from build123d import *

# Parameters (mm, degrees)
ESQUISSE1_W             = 40
ESQUISSE1_H             = 70.5
BOSS_EXTRU_1_DEPTH      = 2
ESQUISSE2_R             = 10
ENL_V_MAT_EXTRU_1_DEPTH = 2
ESQUISSE3_R             = 6.03
ENL_V_MAT_EXTRU_2_DEPTH = 10


with BuildPart() as part:
    # Esquisse1 → Boss.-Extru.1 (new body)
    with BuildSketch(Plane(origin=(0, 0, 0), x_dir=(1, 0, 0), z_dir=(0, 1, 0))):
        with Locations((-5, 5.25)):
            Rectangle(ESQUISSE1_W, ESQUISSE1_H)
        with BuildLine():
            Line((-50, 40.5), (40, 40.5))
            ThreePointArc((40, 40.5), (-5, 85.5), (-50, 40.5))
        make_face()
    extrude(amount=BOSS_EXTRU_1_DEPTH)

    # Esquisse2 → Enlèv. mat.-Extru.1 (cut)
    with BuildSketch(Plane(origin=(0, 2, 0), x_dir=(1, 0, 0), z_dir=(0, 1, 0))):
        with Locations((-5, 40.5)):
            Circle(ESQUISSE2_R)
    extrude(amount=-ENL_V_MAT_EXTRU_1_DEPTH, mode=Mode.SUBTRACT)

    # Esquisse3 → Enlèv. mat.-Extru.2 (cut)
    with BuildSketch(Plane(origin=(0, 0, 0), x_dir=(-1, 0, 0), z_dir=(0, -1, 0))):
        with Locations((5, 75.5)):
            Circle(ESQUISSE3_R)
    extrude(amount=-ENL_V_MAT_EXTRU_2_DEPTH, mode=Mode.SUBTRACT)


solid = part.part
CAD build for the part. Positions are in the model's coordinates, mm. Round coordinates to 2 decimals unless told otherwise and drop trailing zeros. Write each loop counter-clockwise with the first axis right and the second up, starting at its lowest first coordinate (ties: lowest second). Pieces come first, ordered by that corner, then holes.
(1) Slice it at B-B, the plane x = -5. Write the cut outline in (y, z), and give its area (3 significant figures).
(2) Mould opens along X. For faces 1 (the face through (-7.17, 1.01, -30.74)), 2 (the face through (-4.01, 0.99, -85.49)), 3 (the face through (-6, 0, -29)) say: pulls with the +X half, pulls with the -X half, needs draft (parallel to the pull), parting line crosses it, or undercut.
(3) Probe line 1 along Z through (x, y) = (-5, 1); line 2 along Z through (x, y) = (-3.5, 0.75) (3 decimals); line 3 along X through (y, z) = (1.55, -75.5). List the from-to ranges inside material, lowest first.
(4) Slice it at D-D, the plane z = -15. Write the cut outline in (x, y).
(5) Slice it at C-C, the plane z = -75.5. Write the cut outline in (x, y).
(6) Slice it at A-A, the plane y = 1.6. Write the cut outline in (x, z).
(7) Drop flat-ended pins along their axis: P1, Ø1, axis at y = 0.5, z = 2.5, coming from the -X side; P2, Ø1, axis at y = 1.5, z = -73, coming from the +X side; P3, Ø1, axis at x = -38.5, y = 0.5, coming from the +Z side; P4, Ø19.5, axis at x = -5, z = -75.5, coming from the +Y side. Give the stop position or say it passes through.
From the geometry:
1. outline: (0, -85.5) - (2, -85.5) - (2, -81.53) - (0, -81.53) - close; (0, -69.47) - (2, -69.47) - (2, -50.5) - (0, -50.5) - close; (0, -30.5) - (2, -30.5) - (2, 30) - (0, 30) - close
1. area: 167 mm2
2. face 1: undercut
2. face 2: parting line crosses it
2. face 3: needs draft
3. line 1: z = -85.5 to -81.53, -69.47 to -50.5, -30.5 to 30
3. line 2: z = -85.475 to -81.34, -69.66 to -50.387, -30.613 to 30
3. line 3: x = -33.28 to -11.03, 1.03 to 23.28
4. outline: (-25, 0) - (15, 0) - (15, 2) - (-25, 2) - close
5. outline: (-33.28, 0) - (-11.03, 0) - (-11.03, 2) - (-33.28, 2) - close; (1.03, 0) - (23.28, 0) - (23.28, 2) - (1.03, 2) - close
6. outline: (-50, -40.5) arc R45 ccw to (40, -40.5) - (15, -40.5) - (15, 30) - (-25, 30) - (-25, -40.5) - close; hole circle Ø20 at (-5, -40.5); hole circle Ø12.06 at (-5, -75.5)
7. P1: stops at x = -25
7. P2: stops at x = 26.64
7. P3: stops at z = -40.5
7. P4: stops at y = 2
